Here's the drawing with two shaded views (mm, measured from the low corner). I have some questions. Round coordinates to 2 decimals unless told otherwise and drop trailing zeros. Loops run counter-clockwise (first coordinate to the right, second up) from the corner with the lowest first, then second, coordinate; pieces in that order, holes last. Notation, with made-up numbers: (10.5, 89.5) -> (42.5, 89.5) arc R26 ccw to (42.5, 105.5) -> close; hole circle Ø6 at (-16.5, -26.75). An arc over 180 degrees is marked (long way). Write item = value, one per line.
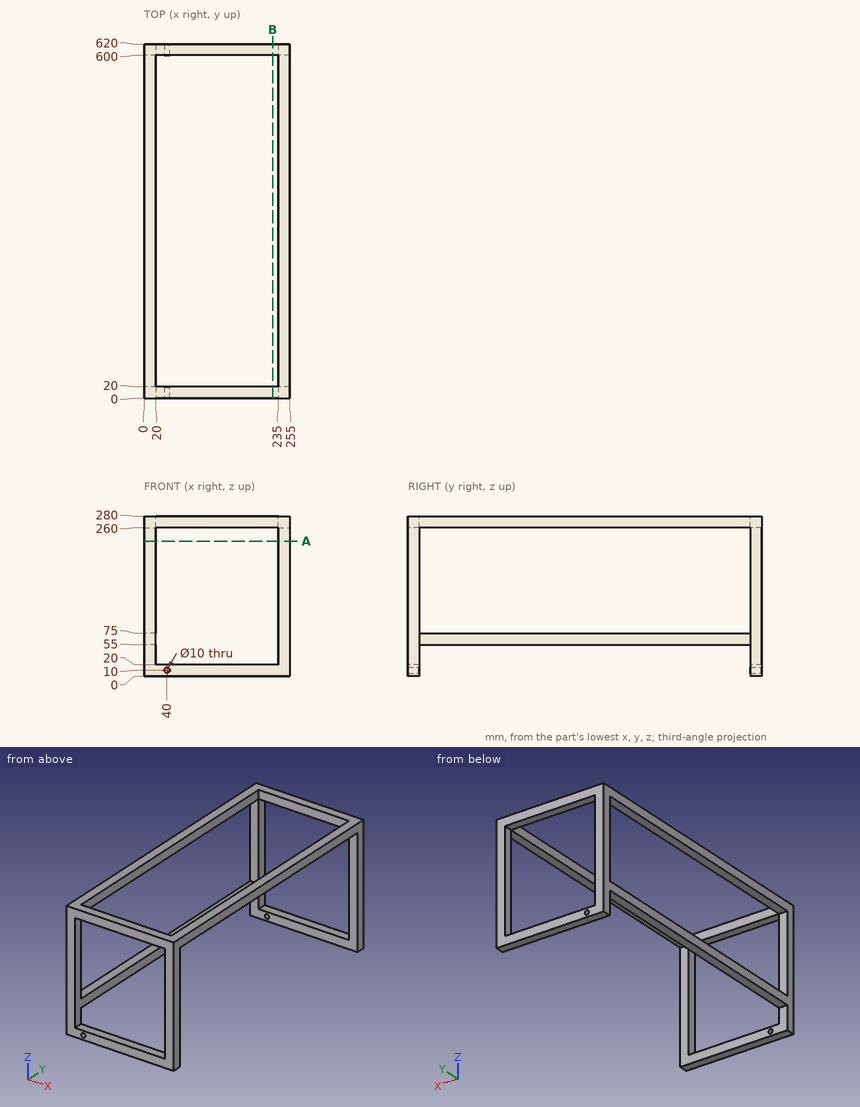
1. Suppose I cut it at A-A, the plane z = 236. List the corners of the cut face in (x, y) for me.
Entries:
outline = (0, 0) -> (20, 0) -> (20, 20) -> (0, 20) -> close; (0, 600) -> (20, 600) -> (20, 620) -> (0, 620) -> close; (235, 0) -> (255, 0) -> (255, 20) -> (235, 20) -> close; (235, 600) -> (255, 600) -> (255, 620) -> (235, 620) -> close
2. I need wall thicknesses on line 1 (Z direction, x = 40, y = 611.5); line 2 (Z direction, x = 240.5, y = 440.5); line 3 (X direction, y = 555, z = 63). Which ranges of each line are inside material? Lowest first, please. Write a range as [from, to].
Entries:
line_1 = [0, 5], [15, 20], [260, 280]
line_2 = [260, 280]
line_3 = [0, 20]
3. I'm going to push flat-ended pins straight in: pin 1 (22 mm diameter, centred on x = 244.5, y = 422.5, fed in from -Z); pin 2 (16 mm diameter, centred on x = 7, y = 343.5, fed in from -Z); pin 3 (8 mm diameter, centred on x = 26, z = 131.5, fed in from -Y). Where does each tip first touch, or does it pass through?
Entries:
pin_1 = 260
pin_2 = 55
pin_3 = through
4. Suppose I cut it at B-B, the plane x = 225. List the corners of the cut face in (y, z) for me.
Entries:
outline = (0, 0) -> (20, 0) -> (20, 20) -> (0, 20) -> close; (0, 260) -> (20, 260) -> (20, 280) -> (0, 280) -> close; (600, 0) -> (620, 0) -> (620, 20) -> (600, 20) -> close; (600, 260) -> (620, 260) -> (620, 280) -> (600, 280) -> close
